```python
from build123d import *

# Parameters (mm, degrees)
SKETCH2_W           = 50
SKETCH2_H           = 90
BOSS_EXTRUDE1_DEPTH = 4
SKETCH3_R           = 6
CUT_EXTRUDE1_DEPTH  = 4
SKETCH4_W           = 50
SKETCH4_H           = 25
CUT_EXTRUDE2_DEPTH  = 10


with BuildPart() as part:
    # Sketch2 → Boss-Extrude1 (new body)
    with BuildSketch(Plane.XY):
        Rectangle(SKETCH2_W, SKETCH2_H)
    extrude(amount=BOSS_EXTRUDE1_DEPTH)

    # Sketch3 → Cut-Extrude1 (cut)
    with BuildSketch(Plane.XY.offset(4)):
        with Locations((0, -25)):
            Circle(SKETCH3_R)
    extrude(amount=-CUT_EXTRUDE1_DEPTH, mode=Mode.SUBTRACT)

    # Sketch4 → Cut-Extrude2 (cut)
    with BuildSketch(Plane.XY.offset(4)):
        with Locations((0, 32.5)):
            Rectangle(SKETCH4_W, SKETCH4_H)
    extrude(amount=-CUT_EXTRUDE2_DEPTH, mode=Mode.SUBTRACT)


solid = part.part
```
The model under review builds one solid part; all positions refer to its coordinate system, in mm. Give positions to 0.01 mm unless a question says otherwise; leave off trailing zeros. Write each loop counter-clockwise with the first axis right and the second up, starting at its lowest first coordinate (ties: lowest second). Pieces come first, ordered by that corner, then holes. Notation, with made-up numbers: (88, 40) - (121, 40) arc R17 cw to (121, 58) - close; hole circle Ø2 at (78.25, 23.5). An arc over 180 degrees is marked (long way). Answer in a Markdown table with one row per item. Add a question column.
1. We need section B-B on y = -25. Write out the cut boundary in (x, z).
2. We need section A-A on x = 0. Write out the cut boundary in (y, z).
3. We need section C-C on z = 2.2. Write out the cut boundary in (x, y).
4. Draft analysis for pull direction X (two halves, no side actions). For faces 1 (the flat face through (0, 20, 2)), 2 (the flat face through (-25, -13, 2)), 3 (the cylindrical face through (-1.301, -30.857, 2.028)), state which applies: +X half, -X half, draft (parallel to the pull), parting line (faces both ways), or undercut.
Ans:
| question | item | result |
|---|---|---|
| 1 | outline | (-25, 0) - (-6, 0) - (-6, 4) - (-25, 4) - close; (6, 0) - (25, 0) - (25, 4) - (6, 4) - close |
| 2 | outline | (-45, 0) - (-31, 0) - (-31, 4) - (-45, 4) - close; (-19, 0) - (20, 0) - (20, 4) - (-19, 4) - close |
| 3 | outline | (-25, -45) - (25, -45) - (25, 20) - (-25, 20) - close; hole circle Ø12 at (0, -25) |
| 4 | face 1 | draft |
| 4 | face 2 | -X half |
| 4 | face 3 | undercut |
